The drawing under review shows one solid part. Ordinate dimensions are in mm from its lowest x, y, z. A direction names the side the tool comes from. Coordinates: 2 decimals unless noted, no trailing zeros. Loops run counter-clockwise (first coordinate to the right, second up) from the corner with the lowest first, then second, coordinate; pieces in that order, holes last. Notation, with made-up numbers: (-11, 75) - (10, 75) arc R35 cw to (10, 107) - close; hole circle Ø4 at (15.25, 69). An arc over 180 degrees is marked (long way). Answer as a JSON object with one key per item and string values. Group by question number.
Item 1: Clearance check with flat-ended pins moving along their axes: pin 1 (20.5 mm diameter, centred on y = 90, z = 23, fed in from -X); pin 2 (4 mm diameter, centred on x = 25, y = 108, fed in from -Z); pin 3 (7.5 mm diameter, centred on x = 65.5, z = 25, fed in from +Y). State where each tip first meets the part, or that it passes through.
Item 2: Tool access review of the marked faces 1, 2 and 3: name each direction out of +Z, -Z, +X, -X, +Y, -Y from which nothing blocks a thin tool from reaching the whole face with its end or side.
Item 3: We need section A-A (z = 10). Give the boundary of the cut face in (x, y).
Item 4: We need section D-D (z = 28.5). Give the boundary of the cut face in (x, y).
Item 5: We need section C-C (y = 28). Give the boundary of the cut face in (x, z).
Item 6: We need section B-B (x = 128). Give the boundary of the cut face in (y, z).
Item 7: To check wall thickness, follow line 1 (Z direction, x = 122.5, y = 108); line 2 (X direction, y = 18, z = 13); line 3 (Y direction, x = 135, z = 24). State the ranges of each line that lie inside material, in increasing order.
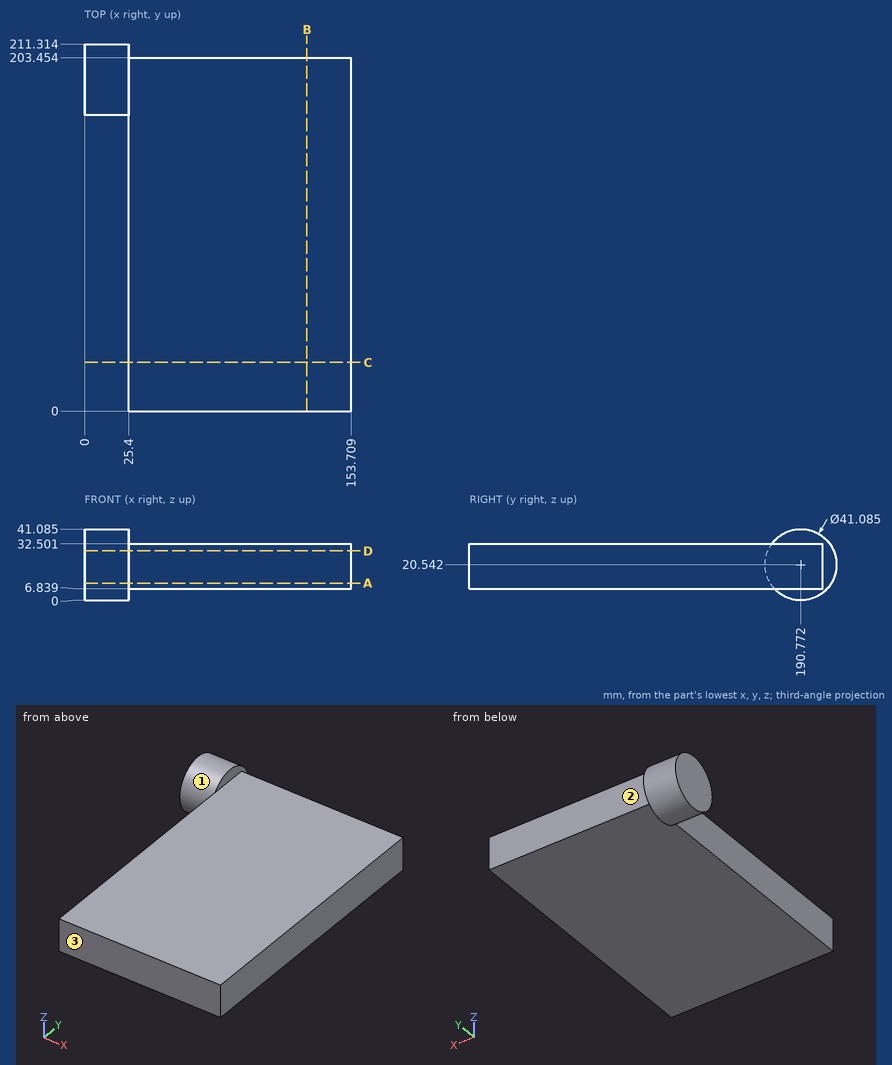
Check sheet entries:
{
 "1": {"pin 1": "stops at x = 25.4", "pin 2": "stops at z = 6.84", "pin 3": "stops at y = 203.45"},
 "2": {"face 1": "-X", "face 2": "+Z, -Z, +X, +Y", "face 3": "+Z, -Z, +X, -X, -Y"},
 "3": {"outline": "(0, 173.14) - (25.4, 173.14) - (25.4, 0) - (153.71, 0) - (153.71, 203.45) - (25.4, 203.45) - (25.4, 208.4) - (0, 208.4) - close"},
 "4": {"outline": "(0, 171.83) - (25.4, 171.83) - (25.4, 0) - (153.71, 0) - (153.71, 203.45) - (25.4, 203.45) - (25.4, 209.71) - (0, 209.71) - close"},
 "5": {"outline": "(25.4, 6.84) - (153.71, 6.84) - (153.71, 32.5) - (25.4, 32.5) - close"},
 "6": {"outline": "(0, 6.84) - (203.45, 6.84) - (203.45, 32.5) - (0, 32.5) - close"},
 "7": {"line 1": "z = 6.84 to 32.5", "line 2": "x = 25.4 to 153.71", "line 3": "y = 0 to 203.45"}
}
